```python
from build123d import *

# Parameters (mm, degrees)
BOSS_EXTRUDE1_DEPTH = 2.54
CUT_EXTRUDE1_REACH  = 4.54
SKETCH2_R           = 1.27
SKETCH2_W           = 5.08
SKETCH2_H           = 5.08
SKETCH2_W_2         = 13.335
SKETCH2_H_2         = 63.5
SKETCH2_W_3         = 12.7
SKETCH2_H_3         = 2.54


with BuildPart() as part:
    # Sketch1 → Boss-Extrude1 (new body)
    with BuildSketch(Plane(origin=(0, 0, 0), x_dir=(1, 0, 0), z_dir=(0, 1, 0))):
        Polygon((-18.034, 63.5), (-18.034, 60.96), (-4.064, 60.96), (-4.064, 63.5), (93.091, 63.5), (93.091, -63.5), (-4.064, -63.5), (-4.064, -60.96), (-18.034, -60.96), (-18.034, -63.5), (-93.091, -63.5), (-93.091, 63.5), align=None)
    extrude(amount=-BOSS_EXTRUDE1_DEPTH)

    # Sketch2 → Cut-Extrude1 (cut, up to next)
    with BuildSketch(Plane(origin=(0, 0, 0), x_dir=(1, 0, 0), z_dir=(0, 1, 0)), mode=Mode.PRIVATE) as cut_extrude1_sk1:
        with Locations((85.471, -12.7)):
            Circle(SKETCH2_R)
    cut_extrude1_tool1 = extrude(cut_extrude1_sk1.sketch, amount=-CUT_EXTRUDE1_REACH, mode=Mode.PRIVATE) & part.part
    add(cut_extrude1_tool1.solids().sort_by_distance((85.471, 0, 12.7))[0], mode=Mode.SUBTRACT)
    # Sketch2 → Cut-Extrude1 (cut, up to next)
    with BuildSketch(Plane(origin=(0, 0, 0), x_dir=(1, 0, 0), z_dir=(0, 1, 0)), mode=Mode.PRIVATE) as cut_extrude1_sk2:
        with Locations((66.421, -12.7)):
            Circle(SKETCH2_R)
    cut_extrude1_tool2 = extrude(cut_extrude1_sk2.sketch, amount=-CUT_EXTRUDE1_REACH, mode=Mode.PRIVATE) & part.part
    add(cut_extrude1_tool2.solids().sort_by_distance((66.421, 0, 12.7))[0], mode=Mode.SUBTRACT)
    # Sketch2 → Cut-Extrude1 (cut, up to next)
    with BuildSketch(Plane(origin=(0, 0, 0), x_dir=(1, 0, 0), z_dir=(0, 1, 0)), mode=Mode.PRIVATE) as cut_extrude1_sk3:
        with Locations((85.471, 12.7)):
            Circle(SKETCH2_R)
    cut_extrude1_tool3 = extrude(cut_extrude1_sk3.sketch, amount=-CUT_EXTRUDE1_REACH, mode=Mode.PRIVATE) & part.part
    add(cut_extrude1_tool3.solids().sort_by_distance((85.471, 0, -12.7))[0], mode=Mode.SUBTRACT)
    # Sketch2 → Cut-Extrude1 (cut, up to next)
    with BuildSketch(Plane(origin=(0, 0, 0), x_dir=(1, 0, 0), z_dir=(0, 1, 0)), mode=Mode.PRIVATE) as cut_extrude1_sk4:
        with Locations((66.421, 12.7)):
            Circle(SKETCH2_R)
    cut_extrude1_tool4 = extrude(cut_extrude1_sk4.sketch, amount=-CUT_EXTRUDE1_REACH, mode=Mode.PRIVATE) & part.part
    add(cut_extrude1_tool4.solids().sort_by_distance((66.421, 0, -12.7))[0], mode=Mode.SUBTRACT)
    # Sketch2 → Cut-Extrude1 (cut, up to next)
    with BuildSketch(Plane(origin=(0, 0, 0), x_dir=(1, 0, 0), z_dir=(0, 1, 0)), mode=Mode.PRIVATE) as cut_extrude1_sk5:
        with Locations((-78.2828, -37.7444)):
            Rectangle(SKETCH2_W, SKETCH2_H)
    cut_extrude1_tool5 = extrude(cut_extrude1_sk5.sketch, amount=-CUT_EXTRUDE1_REACH, mode=Mode.PRIVATE) & part.part
    add(cut_extrude1_tool5.solids().sort_by_distance((-78.2828, 0, 37.7444))[0], mode=Mode.SUBTRACT)
    # Sketch2 → Cut-Extrude1 (cut, up to next)
    with BuildSketch(Plane(origin=(0, 0, 0), x_dir=(1, 0, 0), z_dir=(0, 1, 0)), mode=Mode.PRIVATE) as cut_extrude1_sk6:
        with Locations((-78.2828, 37.7444)):
            Rectangle(SKETCH2_W, SKETCH2_H)
    cut_extrude1_tool6 = extrude(cut_extrude1_sk6.sketch, amount=-CUT_EXTRUDE1_REACH, mode=Mode.PRIVATE) & part.part
    add(cut_extrude1_tool6.solids().sort_by_distance((-78.2828, 0, -37.7444))[0], mode=Mode.SUBTRACT)
    # Sketch2 → Cut-Extrude1 (cut, up to next)
    with BuildSketch(Plane(origin=(0, 0, 0), x_dir=(1, 0, 0), z_dir=(0, 1, 0)), mode=Mode.PRIVATE) as cut_extrude1_sk7:
        with Locations((-13.5509, 0)):
            Rectangle(SKETCH2_W_2, SKETCH2_H_2)
    cut_extrude1_tool7 = extrude(cut_extrude1_sk7.sketch, amount=-CUT_EXTRUDE1_REACH, mode=Mode.PRIVATE) & part.part
    add(cut_extrude1_tool7.solids().sort_by_distance((-13.5509, 0, 0))[0], mode=Mode.SUBTRACT)
    # Sketch2 → Cut-Extrude1 (cut, up to next)
    with BuildSketch(Plane(origin=(0, 0, 0), x_dir=(1, 0, 0), z_dir=(0, 1, 0)), mode=Mode.PRIVATE) as cut_extrude1_sk8:
        with Locations((-11.684, 38.1)):
            Rectangle(SKETCH2_W_3, SKETCH2_H_3)
    cut_extrude1_tool8 = extrude(cut_extrude1_sk8.sketch, amount=-CUT_EXTRUDE1_REACH, mode=Mode.PRIVATE) & part.part
    add(cut_extrude1_tool8.solids().sort_by_distance((-11.684, 0, -38.1))[0], mode=Mode.SUBTRACT)
    # Sketch2 → Cut-Extrude1 (cut, up to next)
    with BuildSketch(Plane(origin=(0, 0, 0), x_dir=(1, 0, 0), z_dir=(0, 1, 0)), mode=Mode.PRIVATE) as cut_extrude1_sk9:
        with Locations((-11.684, -38.1)):
            Rectangle(SKETCH2_W_3, SKETCH2_H_3)
    cut_extrude1_tool9 = extrude(cut_extrude1_sk9.sketch, amount=-CUT_EXTRUDE1_REACH, mode=Mode.PRIVATE) & part.part
    add(cut_extrude1_tool9.solids().sort_by_distance((-11.684, 0, 38.1))[0], mode=Mode.SUBTRACT)
    # Sketch2 → Cut-Extrude1 (cut, up to next)
    with BuildSketch(Plane(origin=(0, 0, 0), x_dir=(1, 0, 0), z_dir=(0, 1, 0)), mode=Mode.PRIVATE) as cut_extrude1_sk10:
        with Locations((67.183, -29.972)):
            Rectangle(SKETCH2_W, SKETCH2_H)
    cut_extrude1_tool10 = extrude(cut_extrude1_sk10.sketch, amount=-CUT_EXTRUDE1_REACH, mode=Mode.PRIVATE) & part.part
    add(cut_extrude1_tool10.solids().sort_by_distance((67.183, 0, 29.972))[0], mode=Mode.SUBTRACT)
    # Sketch2 → Cut-Extrude1 (cut, up to next)
    with BuildSketch(Plane(origin=(0, 0, 0), x_dir=(1, 0, 0), z_dir=(0, 1, 0)), mode=Mode.PRIVATE) as cut_extrude1_sk11:
        with Locations((-33.4772, 37.7444)):
            Rectangle(SKETCH2_W, SKETCH2_H)
    cut_extrude1_tool11 = extrude(cut_extrude1_sk11.sketch, amount=-CUT_EXTRUDE1_REACH, mode=Mode.PRIVATE) & part.part
    add(cut_extrude1_tool11.solids().sort_by_distance((-33.4772, 0, -37.7444))[0], mode=Mode.SUBTRACT)
    # Sketch2 → Cut-Extrude1 (cut, up to next)
    with BuildSketch(Plane(origin=(0, 0, 0), x_dir=(1, 0, 0), z_dir=(0, 1, 0)), mode=Mode.PRIVATE) as cut_extrude1_sk12:
        with Locations((-33.3502, -37.7444)):
            Rectangle(SKETCH2_W, SKETCH2_H)
    cut_extrude1_tool12 = extrude(cut_extrude1_sk12.sketch, amount=-CUT_EXTRUDE1_REACH, mode=Mode.PRIVATE) & part.part
    add(cut_extrude1_tool12.solids().sort_by_distance((-33.3502, 0, 37.7444))[0], mode=Mode.SUBTRACT)
    # Sketch2 → Cut-Extrude1 (cut, up to next)
    with BuildSketch(Plane(origin=(0, 0, 0), x_dir=(1, 0, 0), z_dir=(0, 1, 0)), mode=Mode.PRIVATE) as cut_extrude1_sk13:
        with Locations((67.183, 29.972)):
            Rectangle(SKETCH2_W, SKETCH2_H)
    cut_extrude1_tool13 = extrude(cut_extrude1_sk13.sketch, amount=-CUT_EXTRUDE1_REACH, mode=Mode.PRIVATE) & part.part
    add(cut_extrude1_tool13.solids().sort_by_distance((67.183, 0, -29.972))[0], mode=Mode.SUBTRACT)
    # Sketch2 → Cut-Extrude1 (cut, up to next)
    with BuildSketch(Plane(origin=(0, 0, 0), x_dir=(1, 0, 0), z_dir=(0, 1, 0)), mode=Mode.PRIVATE) as cut_extrude1_sk14:
        with Locations((14.097, 29.972)):
            Rectangle(SKETCH2_W, SKETCH2_H)
    cut_extrude1_tool14 = extrude(cut_extrude1_sk14.sketch, amount=-CUT_EXTRUDE1_REACH, mode=Mode.PRIVATE) & part.part
    add(cut_extrude1_tool14.solids().sort_by_distance((14.097, 0, -29.972))[0], mode=Mode.SUBTRACT)
    # Sketch2 → Cut-Extrude1 (cut, up to next)
    with BuildSketch(Plane(origin=(0, 0, 0), x_dir=(1, 0, 0), z_dir=(0, 1, 0)), mode=Mode.PRIVATE) as cut_extrude1_sk15:
        with Locations((14.097, -29.972)):
            Rectangle(SKETCH2_W, SKETCH2_H)
    cut_extrude1_tool15 = extrude(cut_extrude1_sk15.sketch, amount=-CUT_EXTRUDE1_REACH, mode=Mode.PRIVATE) & part.part
    add(cut_extrude1_tool15.solids().sort_by_distance((14.097, 0, 29.972))[0], mode=Mode.SUBTRACT)


solid = part.part
```
The listing builds one solid part. Answer for the finished solid, in the listing's coordinates (mm). Coordinates: 2 decimals unless noted, no trailing zeros. Loops run counter-clockwise (first coordinate to the right, second up) from the corner with the lowest first, then second, coordinate; pieces in that order, holes last. Notation, with made-up numbers: (-4, 11) - (33, 11) arc R25 ccw to (33, 25) - close; hole circle Ø8 at (20.25, 3). An arc over 180 degrees is marked (long way). Write item = value, one per line.
1) Section A-A (z = -24) is taken. Determine the outline of the cut face in (x, y).
Responses:
outline = (-93.09, -2.54) - (-20.22, -2.54) - (-20.22, 0) - (-93.09, 0) - close; (-6.88, -2.54) - (93.09, -2.54) - (93.09, 0) - (-6.88, 0) - close
2) Each of these flat-tipped pins is pushed along its axis until it touches: P1, Ø8, axis at x = -9, z = -23, coming from the +Y side; P2, Ø1.3, axis at x = -9, y = -2, coming from the -Z side; P3, Ø0.8, axis at x = -11.5, y = -1, coming from the +Z side. Where does it stop, or does it pass through?
Responses:
P1 = 0
P2 = -60.96
P3 = 60.96
3) Section C-C (y = -1.2) is taken. Count the separate pieces of the cut face and the enclosed holes in it, plus the area to 3 significant figures.
Responses:
separate_pieces = 1
enclosed_holes = 15
area = 22,400 mm^2
4) Section B-B (x = -10.5) is taken. Determine the outline of the cut face in (y, z).
Responses:
outline = (-2.54, -60.96) - (0, -60.96) - (0, -39.37) - (-2.54, -39.37) - close; (-2.54, -36.83) - (0, -36.83) - (0, -31.75) - (-2.54, -31.75) - close; (-2.54, 31.75) - (0, 31.75) - (0, 36.83) - (-2.54, 36.83) - close; (-2.54, 39.37) - (0, 39.37) - (0, 60.96) - (-2.54, 60.96) - close
5) Find the intervals of material crossed by line 1 along Z through (x, y) = (15.5, -0.4); line 2 along X through (y, z) = (-0.45, -12.7); line 3 along Z through (x, y) = (-6, -2.4), in increasing order.
Responses:
line_1 = -63.5 to -32.51, -27.43 to 27.43, 32.51 to 63.5
line_2 = -93.09 to -20.22, -6.88 to 65.15, 67.69 to 84.2, 86.74 to 93.09
line_3 = -60.96 to -39.37, -36.83 to 36.83, 39.37 to 60.96
